from build123d import *

# Parameters (mm, degrees)
F0_R     = 16.935
F1_DEPTH = 20.5
F2_R     = 12.75
F3_DEPTH = 5.5
F4_R     = 11.1125
F5_DEPTH = 40.132


with BuildPart() as f1:
    # F0 (on Top) → F1 (new body)
    with BuildSketch(Plane.XY):
        Circle(F0_R)
    extrude(amount=F1_DEPTH)

    # F2 (on face) → F3 (join)
    with BuildSketch(Plane.XY.offset(20.5)):
        with Locations((0, 0.00292)):
            Circle(F2_R)
    extrude(amount=F3_DEPTH)

    # F4 (on face) → F5 (cut)
    with BuildSketch(Plane.XY.offset(26)):
        Circle(F4_R)
    extrude(amount=-F5_DEPTH, mode=Mode.SUBTRACT)


solid = f1.part
The listing builds one solid part. Answer for the finished solid, in the listing's coordinates (mm). A direction names the side the tool comes from. Round coordinates to 2 decimals unless told otherwise and drop trailing zeros. Write each loop counter-clockwise with the first axis right and the second up, starting at its lowest first coordinate (ties: lowest second). Pieces come first, ordered by that corner, then holes. Notation, with made-up numbers: M 7,-12.5 L 23,-12.5 A12 ccw 23,0.5 Z; hole C 71.5,75 d7. An arc over 180 degrees is marked long. Write each question's results on one line, items separated by ' | '. Start each with the question number.
Item 1: Find section D-D on y = 15.5. Write down the section's boundary in (x, z).
Item 2: Find section B-B on y = -10. Write down the section's boundary in (x, z).
Item 3: Find section A-A on x = -1. Write down the section's boundary in (y, z).
Item 4: The mould has two halves that part along X. Classify faces 1 (the cylindrical face through (10.6, 3.34, 13.18)), 2 (the flat face through (0.9, 11.4, 26)), 3 (the cylindrical face through (-10.118, -7.755, 23.212)): +X half, -X half, draft (parallel to the pull), parting line (faces both ways), or undercut.
Item 5: Find section C-C on z = 13.5. Write down the section's boundary in (x, y) (1 decimal), and give its area (3 significant figures).
Item 6: Given pin 1 Ø6 at (x, y) = (-12.5, -10) entering from +Z; pin 2 Ø1 at (y, z) = (10, 5) entering from +X; pin 3 Ø3 at (y, z) = (10, 20) entering from +X; pin 4 Ø3 at (x, y) = (-8, -2) entering from +Z, each flat-ended and moving along its own axis, determine where each tip first touches the part or whether it passes through.
Item 7: Straight lines are drawn through the part: probe 1 along Y at (x, z) = (0, 6.5) (1 decimal); probe 2 along Z at (x, y) = (-9, -13); probe 3 along Y at (x, z) = (-3, 5). For each, find the intervals that lie inside material, in ascending order.
Item 8: Which of the six approach directions +Z, -Z, +X, -X, +Y, -Y give full straight-line access (tool end or side, diameter ignored) to faces 4 (the flat face through (2, 13, 20.5)), 5 (the flat face through (4, -11, 0))?
Answer block:
1) outline: M -6.82,0 L 6.82,0 L 6.82,20.5 L -6.82,20.5 Z
2) outline: M -13.67,0 L -4.85,0 L -4.85,26 L -7.91,26 L -7.91,20.5 L -13.67,20.5 Z; M 4.85,0 L 13.67,0 L 13.67,20.5 L 7.91,20.5 L 7.91,26 L 4.85,26 Z
3) outline: M -16.91,0 L -11.07,0 L -11.07,26 L -12.71,26 L -12.71,20.5 L -16.91,20.5 Z; M 11.07,0 L 16.91,0 L 16.91,20.5 L 12.71,20.5 L 12.71,26 L 11.07,26 Z
4) face 1: undercut | face 2: draft | face 3: parting line
5) outline: C 0,0 d33.9; hole C 0,0 d22.2 | area: 513 mm²
6) pin 1: stops at z = 20.5 | pin 2: stops at x = 14.02 | pin 3: stops at x = 14.65 | pin 4: passes through
7) probe 1: y = -16.9 to -11.1, 11.1 to 16.9 | probe 2: z = 0 to 20.5 | probe 3: y = -16.67 to -10.7, 10.7 to 16.67
8) face 4: +Z | face 5: -Z, +X, -X, +Y, -Y
